from build123d import *

# Parameters (mm, degrees)
BOSS_EXTRUDE1_DEPTH      = 3.556
BOSS_EXTRUDE1_DEPTH_BACK = 3.556
SKETCH2_R                = 18.7325
BOSS_EXTRUDE2_DEPTH      = 6.9215
BOSS_EXTRUDE2_DEPTH_BACK = 6.9215
SKETCH4_R                = 7.9375
FILLET1_R                = 6.35
CUT_EXTRUDE1_DEPTH       = 30.890496174
CUT_EXTRUDE1_DEPTH_BACK  = 30.890496174
SKETCH5_R                = 0.79375


with BuildPart() as part:
    # Sketch2 → Boss-Extrude1 (new, two sides: drawn at the far end of the back side and taken through both)
    with BuildSketch(Plane.XY.offset(-BOSS_EXTRUDE1_DEPTH_BACK)):
        Circle(SKETCH2_R)
    extrude(amount=BOSS_EXTRUDE1_DEPTH + BOSS_EXTRUDE1_DEPTH_BACK)

    # Sketch3 → Cut-Revolve1 (revolve, cut)
    with BuildSketch(Plane(origin=(0, 0, 0), x_dir=(0, 0, -1), z_dir=(1, 0, 0)), mode=Mode.PRIVATE) as cut_revolve1_sk:
        with BuildLine():
            Line((-2.2225, 16.51), (-2.2225, 20.955))
            Line((-2.2225, 20.955), (2.2225, 20.955))
            Line((2.2225, 20.955), (2.2225, 16.51))
            ThreePointArc((2.2225, 16.51), (0, 14.2875), (-2.2225, 16.51))
        make_face()
    revolve(cut_revolve1_sk.sketch.rotate(Axis((0, 0, 3.556), (0, 0, -1)), 90), axis=Axis((0, 0, 3.556), (0, 0, -1)), mode=Mode.SUBTRACT)

    # Sketch4 → Boss-Extrude2 (add, two sides: drawn at the far end of the back side and taken through both)
    with BuildSketch(Plane.XY.offset(-BOSS_EXTRUDE2_DEPTH_BACK)):
        Circle(SKETCH4_R)
    extrude(amount=BOSS_EXTRUDE2_DEPTH + BOSS_EXTRUDE2_DEPTH_BACK)

    # Fillet1
    # the kernel refuses this fillet: 6.35 mm, written as the material it adds along each edge
    with BuildSketch(Plane(origin=(0, 0, 3.556), x_dir=(1, 0, 0), z_dir=(0, 1, 0))) as fillet1_piece_1:
        with BuildLine():
            CenterArc((13.542431735, -6.35), FILLET1_R, 90, 61.965703465)
            Line((7.9375, -3.3655), (7.825401365, -3.30581))
            ThreePointArc((7.825401365, -3.30581), (7.8105, -1.68275), (7.8105, 0))
            Line((7.8105, 0), (7.9375, 0.127))
            Line((7.9375, 0.127), (13.542431735, 0.127))
            Line((13.542431735, 0.127), (13.542431735, 0))
        make_face()
    revolve(axis=Axis((0, 0, 3.556), (0, 0, -1)))
    with BuildSketch(Plane(origin=(0, 0, -3.556), x_dir=(1, 0, 0), z_dir=(0, -1, 0))) as fillet1_piece_2:
        with BuildLine():
            CenterArc((13.542431735, -6.35), FILLET1_R, 90, 61.965703465)
            Line((7.9375, -3.3655), (7.825401365, -3.30581))
            ThreePointArc((7.825401365, -3.30581), (7.8105, -1.68275), (7.8105, 0))
            Line((7.8105, 0), (7.9375, 0.127))
            Line((7.9375, 0.127), (13.542431735, 0.127))
            Line((13.542431735, 0.127), (13.542431735, 0))
        make_face()
    revolve(axis=Axis((0, 0, -3.556), (0, 0, 1)))

    # Sketch5 → Cut-Extrude1 (cut, two sides: drawn at the far end of the back side and taken through both)
    with BuildSketch(Plane.XY.offset(6.9215).offset(-CUT_EXTRUDE1_DEPTH_BACK)):
        Circle(SKETCH5_R)
    extrude(amount=CUT_EXTRUDE1_DEPTH + CUT_EXTRUDE1_DEPTH_BACK, mode=Mode.SUBTRACT)


solid = part.part
Build history of the part. All positions in model axes, mm. A direction names the side the tool comes from. Coordinates: 2 decimals unless noted, no trailing zeros. Order: outer loops, then holes, each group sorted by start corner. A loop starts at its lowest first (then second) coordinate and runs counter-clockwise, first axis right, second up. Notation, with made-up numbers: (29, 84) - (78, 84) arc R26 ccw to (78, 111) - close; hole circle Ø4 at (59.5, 22.25). An arc over 180 degrees is marked (long way). Put each result on its own line as item: value.
1. Saw through at C-C (z = -1.5). Write the cut outline in (x, y).
Answer sheet:
outline: circle Ø29.74 at (0, 0); hole circle Ø1.59 at (0, 0)
2. Pull direction X, two halves, no side cores. Call faces 1 (the face through (0, 17, -2.222)), 2 (the face through (-14.865, -11.398, 2.88)), 3 (the face through (-0.172, -0.775, -0.097)): pulls with the +X half, pulls with the -X half, needs draft (parallel to the pull), parting line crosses it, or undercut.
Answer sheet:
face 1: needs draft
face 2: parting line crosses it
face 3: undercut
3. Saw through at D-D (z = 2.75). Write the cut outline in (x, y) (1 decimal), and give its area (3 significant figures).
Answer sheet:
outline: circle Ø37.5 at (0, 0); hole circle Ø1.6 at (0, 0)
area: 1,100 mm^2
4. Tool access for faces 4 (the face through (10, 10, 3.556)), 5 (the face through (2, 0, 6.922)), 6 (the face through (10, 10, -3.556)), 7 (the face through (0, 17, 2.222)), 8 (the face through (-14.865, -11.398, -2.899)): list every direction of +Z, -Z, +X, -X, +Y, -Y with a clear straight run to the whole face (end or side of a thin tool).
Answer sheet:
face 4: +Z
face 5: +Z, +X, -X, +Y, -Y
face 6: -Z
face 7: none
face 8: +Z, -Z
5. Drop flat-ended pins along their axis: P1, Ø11, axis at x = 6, y = -6.5, coming from the +Z side; P2, Ø8, axis at x = -12.5, y = 9.5, coming from the -Z side; P3, Ø4, axis at x = 5, z = 3.5, coming from the -Y side; P4, Ø12, axis at x = -2, y = -14, coming from the -Z side. Give the stop position or say it passes through.
Answer sheet:
P1: stops at z = 6.92
P2: stops at z = -3.83
P3: stops at y = -18.49
P4: stops at z = -6.57
6. Probe line 1 along Z through (x, y) = (-13, -12); line 2 along Y through (x, z) = (0, 3); line 3 along Y through (x, z) = (0, -2). List the from-to ranges inside material, lowest first. Write a range as [from, to].
Answer sheet:
line 1: z = [-3.56, -2.22], [2.22, 3.56]
line 2: y = [-18.73, -0.79], [0.79, 18.73]
line 3: y = [-15.54, -0.79], [0.79, 15.54]
